from build123d import *

# Parameters (mm, degrees)
SKETCH_1_W             = 35
SKETCH_1_H             = 70
SKETCH_1_R             = 2.6
EXTRUDE_505_DEPTH      = 3
SKETCH_2_R             = 2.1
CUT_EXTRUDE_M4_DEPTH   = 3
SKETCH_3_R             = 2.6
EXTRUDE_967_DEPTH      = 3
SKETCH_4_R             = 2.1
CUT_EXTRUDE_1312_DEPTH = 4
SKETCH_5_W             = 49
SKETCH_5_H             = 70
EXTRA_DEPTH            = 3
SKETCH_6_R             = 2.1
CUT_EXTRUDE_2055_DEPTH = 10
SKETCH_7_R             = 2.1
ETRA_DEPTH             = 10
SKETCH_10_R            = 1.6
SKETCH_10_R_2          = 3.5
CUT_EXTRUDE_3548_DEPTH = 4
FILLET_5_0_R           = 5
SKETCH_12_R            = 2.1
EXTRUDE_1_DEPTH        = 3
SKETCH_13_R            = 1.5
CUT_EXTRUDE_1_DEPTH    = 4
SKETCH_15_W            = 32.658399477
SKETCH_15_H            = 70
CUT_EXTRUDE_4_DEPTH    = 4
FILLET_6_R             = 5
SKETCH_16_R            = 1.6
SKETCH_16_R_2          = 1.603432059
EXTRUDE_2_DEPTH        = 3
SKETCH_17_R            = 2.5
CUT_EXTRUDE_5_DEPTH    = 4
SKETCH_18_R            = 1.5
EXTRUDE_3_DEPTH        = 3
SKETCH_19_R            = 1.2
CUT_EXTRUDE_6_DEPTH    = 4
SKETCH_20_R            = 2.1
SKETCH_20_R_2          = 1.6
SKETCH_20_R_3          = 2.55820294
EXTRUDE_4_DEPTH        = 3
SKETCH_22_R            = 3.5
SKETCH_22_R_2          = 2.5
EXTRUDE_5_DEPTH        = 3
SKETCH_25_R            = 2.5
CUT_EXTRUDE_9_DEPTH    = 4
SKETCH_26_R            = 2.6
SKETCH_26_R_2          = 1.6
CUT_EXTRUDE_10_DEPTH   = 4


with BuildPart() as part:
    # 草图1 → Extrude 505 (new body)
    with BuildSketch(Plane(origin=(0, 0, 0), x_dir=(1, 0, 0), z_dir=(0, 1, 0))):
        Rectangle(SKETCH_1_W, SKETCH_1_H)
        with Locations((-7.5, 22.5)):
            Circle(SKETCH_1_R, mode=Mode.SUBTRACT)
        with Locations((-7.5, 0)):
            Circle(SKETCH_1_R, mode=Mode.SUBTRACT)
        with Locations((-7.5, -22.5)):
            Circle(SKETCH_1_R, mode=Mode.SUBTRACT)
        with Locations((-7.5, 10)):
            Circle(SKETCH_1_R, mode=Mode.SUBTRACT)
        with Locations((-7.5, -10)):
            Circle(SKETCH_1_R, mode=Mode.SUBTRACT)
    extrude(amount=EXTRUDE_505_DEPTH)

    # 草图2 → M4铝柱 (cut)
    with BuildSketch(Plane(origin=(0, 3, 0), x_dir=(1, 0, 0), z_dir=(0, 1, 0))):
        with Locations((10, 0)):
            Circle(SKETCH_2_R)
    extrude(amount=-CUT_EXTRUDE_M4_DEPTH, mode=Mode.SUBTRACT)

    # 草图3 → Extrude 967 (add, through all)
    with BuildSketch(Plane(origin=(0, 3, 0), x_dir=(1, 0, 0), z_dir=(0, 1, 0))):
        with Locations((-7.5, -10)):
            Circle(SKETCH_3_R)
        with Locations((-7.5, 10)):
            Circle(SKETCH_3_R)
    extrude(amount=-EXTRUDE_967_DEPTH)

    # 草图4 → Cut-Extrude 1312 (cut, through all)
    with BuildSketch(Plane(origin=(0, 3, 0), x_dir=(1, 0, 0), z_dir=(0, 1, 0))):
        with Locations((10, 22.5)):
            Circle(SKETCH_4_R)
        with Locations((10, -22.5)):
            Circle(SKETCH_4_R)
    extrude(amount=-CUT_EXTRUDE_1312_DEPTH, mode=Mode.SUBTRACT)

    # 草图5 → EXTRA (add, through all)
    with BuildSketch(Plane(origin=(0, 3, 0), x_dir=(1, 0, 0), z_dir=(0, 1, 0))):
        with Locations((-42, 0)):
            Rectangle(SKETCH_5_W, SKETCH_5_H)
    extrude(amount=-EXTRA_DEPTH)

    # 草图6 → Cut-Extrude 2055 (cut)
    with BuildSketch(Plane(origin=(0, 3, 0), x_dir=(1, 0, 0), z_dir=(0, 1, 0))):
        with Locations((-44.5, 0)):
            Circle(SKETCH_6_R)
        with Locations((-36.5, 0)):
            Circle(SKETCH_6_R)
    extrude(amount=-CUT_EXTRUDE_2055_DEPTH, mode=Mode.SUBTRACT)

    # 草图7 → ETRA铝柱 (cut)
    with BuildSketch(Plane(origin=(0, 3, 0), x_dir=(1, 0, 0), z_dir=(0, 1, 0))):
        with Locations((-60, 17.5)):
            Circle(SKETCH_7_R)
        with Locations((-60, -17.5)):
            Circle(SKETCH_7_R)
    extrude(amount=-ETRA_DEPTH, mode=Mode.SUBTRACT)

    # 草图10 → Cut-Extrude 3548 (cut, through all)
    with BuildSketch(Plane.XZ):
        with Locations((-43.5, -21.25)):
            Circle(SKETCH_10_R)
        with Locations((-21.5, -31.75)):
            Circle(SKETCH_10_R)
        with Locations((-43.5, -31.75)):
            Circle(SKETCH_10_R)
        with Locations((-43.5, 21.25)):
            Circle(SKETCH_10_R)
        with Locations((-21.5, 31.75)):
            Circle(SKETCH_10_R)
        with Locations((-43.5, 31.75)):
            Circle(SKETCH_10_R)
        with Locations((-21.5, 21.25)):
            Circle(SKETCH_10_R_2)
        with Locations((-21.5, -21.25)):
            Circle(SKETCH_10_R_2)
    extrude(amount=-CUT_EXTRUDE_3548_DEPTH, mode=Mode.SUBTRACT)

    # 圆角5.0
    fillet_5_0_edges = [part.edges().sort_by_distance(p)[0] for p in [
        (-66.5, 1.5, 35),
        (-66.5, 1.5, -35),
        (17.5, 1.5, 35),
        (17.5, 1.5, -35),
    ]]
    fillet(fillet_5_0_edges, radius=FILLET_5_0_R)

    # 草图12 → 凸台-拉伸1 (add)
    with BuildSketch(Plane(origin=(0, 3, 0), x_dir=(1, 0, 0), z_dir=(0, 1, 0))):
        with Locations((-36.5, 0)):
            Circle(SKETCH_12_R)
        with Locations((-44.5, 0)):
            Circle(SKETCH_12_R)
    extrude(amount=-EXTRUDE_1_DEPTH)

    # 草图13 → 切除-拉伸1 (cut, through all)
    with BuildSketch(Plane(origin=(0, 3, 0), x_dir=(1, 0, 0), z_dir=(0, 1, 0))):
        with Locations((-52.499999555, 1.426e-06)):
            Circle(SKETCH_13_R)
        with Locations((-28.499999555, 1.44e-06)):
            Circle(SKETCH_13_R)
    extrude(amount=-CUT_EXTRUDE_1_DEPTH, mode=Mode.SUBTRACT)

    # 草图15 → 切除-拉伸4 (cut, through all)
    with BuildSketch(Plane(origin=(0, 3, 0), x_dir=(1, 0, 0), z_dir=(0, 1, 0))):
        with Locations((2.675548589, 0)):
            Rectangle(SKETCH_15_W, SKETCH_15_H)
    extrude(amount=-CUT_EXTRUDE_4_DEPTH, mode=Mode.SUBTRACT)

    # 圆角6
    fillet_6_edges = [part.edges().sort_by_distance(p)[0] for p in [
        (-13.653651149, 1.5, -35),
        (-13.653651149, 1.5, 35),
    ]]
    fillet(fillet_6_edges, radius=FILLET_6_R)

    # 草图16 → 凸台-拉伸2 (add)
    with BuildSketch(Plane.XZ):
        with Locations((-21.5, 31.75)):
            Circle(SKETCH_16_R)
        with Locations((-21.5, -31.75)):
            Circle(SKETCH_16_R_2)
    extrude(amount=-EXTRUDE_2_DEPTH)

    # 草图17 → 切除-拉伸5 (cut, through all)
    with BuildSketch(Plane(origin=(0, 3, 0), x_dir=(1, 0, 0), z_dir=(0, 1, 0))):
        with Locations((-23.393651149, -30)):
            Circle(SKETCH_17_R)
        with Locations((-24.763651149, 30)):
            Circle(SKETCH_17_R)
    extrude(amount=-CUT_EXTRUDE_5_DEPTH, mode=Mode.SUBTRACT)

    # 草图18 → 凸台-拉伸3 (add)
    with BuildSketch(Plane.XZ):
        with Locations((-52.499999555, -1.426e-06)):
            Circle(SKETCH_18_R)
        with Locations((-28.499999555, -1.44e-06)):
            Circle(SKETCH_18_R)
    extrude(amount=-EXTRUDE_3_DEPTH)

    # 草图19 → 切除-拉伸6 (cut, through all)
    with BuildSketch(Plane.XZ):
        with Locations((-54.153651149, -2.448052536)):
            Circle(SKETCH_19_R)
        with Locations((-34.153651149, -2.448052536)):
            Circle(SKETCH_19_R)
    extrude(amount=-CUT_EXTRUDE_6_DEPTH, mode=Mode.SUBTRACT)

    # 草图20 → 凸台-拉伸4 (add)
    with BuildSketch(Plane.XZ):
        with Locations((-60, 17.5)):
            Circle(SKETCH_20_R)
        with Locations((-43.5, 21.25)):
            Circle(SKETCH_20_R_2)
        with Locations((-43.653651149, 31.685692809)):
            Circle(SKETCH_20_R_3)
    extrude(amount=-EXTRUDE_4_DEPTH)

    # 草图22 → 凸台-拉伸5 (add)
    with BuildSketch(Plane(origin=(0, 0, 0), x_dir=(-1, 0, 0), z_dir=(0, -1, 0))):
        with Locations((21.5, 21.25)):
            Circle(SKETCH_22_R)
        with Locations((24.763651149, 30)):
            Circle(SKETCH_22_R_2)
    extrude(amount=-EXTRUDE_5_DEPTH)

    # 草图25 → 切除-拉伸9 (cut, through all)
    with BuildSketch(Plane(origin=(0, 3, 0), x_dir=(1, 0, 0), z_dir=(0, 1, 0))):
        with Locations((-23.393651149, 25.376236088)):
            Circle(SKETCH_25_R)
    extrude(amount=-CUT_EXTRUDE_9_DEPTH, mode=Mode.SUBTRACT)

    # 草图26 → 切除-拉伸10 (cut, through all)
    with BuildSketch(Plane.XZ):
        with Locations((-55.153651029, 27.841992404)):
            Circle(SKETCH_26_R)
        with Locations((-23.393651149, -25.376236088)):
            Circle(SKETCH_26_R)
        with Locations((-23.393651149, 30)):
            Circle(SKETCH_26_R)
        with Locations((-55.153651029, 10.96736207)):
            Circle(SKETCH_26_R)
        with Locations((-54.153651149, -2.448052536)):
            Circle(SKETCH_26_R_2)
        with Locations((-34.153651149, -2.448052536)):
            Circle(SKETCH_26_R_2)
    extrude(amount=-CUT_EXTRUDE_10_DEPTH, mode=Mode.SUBTRACT)


solid = part.part
CAD build for the part. Positions are in the model's coordinates, mm. Coordinates: 2 decimals unless noted, no trailing zeros. Order: outer loops, then holes, each group sorted by start corner. A loop starts at its lowest first (then second) coordinate and runs counter-clockwise, first axis right, second up.
Item 1: Two-plate mould, pull along Z, no slides. Class faces 1 (the face through (-15.079, 1.479, 33.496)), 2 (the face through (-32.628, 1.479, -1.967)), 3 (the face through (-40, 3, 0)): +Z half, -Z half, draft (parallel to the pull), parting line (faces both ways), or undercut.
Check sheet entries:
face 1: +Z half
face 2: undercut
face 3: draft
Item 2: Drill centre lines: L1, parallel to Z at x = -43.5, y = 1.65; L2, parallel to Z at x = -57, y = 0.4; L3, parallel to Z at x = -33, y = 1.5. Where is each one in solid material? Low to high.
Check sheet entries:
L1: z = -35 to -33.35, -30.15 to -22.85, -19.65 to 35
L2: z = -35 to 9.14, 12.8 to 26.01, 29.67 to 35
L3: z = -35 to -3.56, -1.34 to 35
Item 3: Band-saw the part on A-A on z = -21.25. List the corners of the cut face in (x, y), plus the area to 3 significant figures.
Check sheet entries:
outline: (-66.5, 0) - (-45.1, 0) - (-45.1, 3) - (-66.5, 3) - close; (-41.9, 0) - (-13.65, 0) - (-13.65, 3) - (-41.9, 3) - close
area: 149 mm2
Item 4: Band-saw the part on D-D on x = -21.5. List the corners of the cut face in (y, z), plus the area to 3 significant figures.
Check sheet entries:
outline: (0, -35) - (3, -35) - (3, -27.16) - (0, -27.16) - close; (0, -23.59) - (3, -23.59) - (3, 17.75) - (0, 17.75) - close; (0, 24.75) - (3, 24.75) - (3, 28.22) - (0, 28.22) - close; (0, 31.78) - (3, 31.78) - (3, 35) - (0, 35) - close
area: 168 mm2
Item 5: Band-saw the part on C-C on y = 0.45. Give the number of separate pieces and of enclosed holes in the cut face, plus the area to 3 significant figures.
Check sheet entries:
separate pieces: 1
enclosed holes: 10
area: 3,510 mm2
Item 6: Band-saw the part on B-B on x = -60. List the corners of the cut face in (y, z), plus the area to 3 significant figures.
Check sheet entries:
outline: (0, -35) - (3, -35) - (3, -19.6) - (0, -19.6) - close; (0, -15.4) - (3, -15.4) - (3, 35) - (0, 35) - close
area: 197 mm2
